Build history of the part. All positions in model axes, mm. A direction names the side the tool comes from. Give positions to 0.01 mm unless a question says otherwise; leave off trailing zeros. Order: outer loops, then holes, each group sorted by start corner. A loop starts at its lowest first (then second) coordinate and runs counter-clockwise, first axis right, second up. Notation, with made-up numbers: (58.25, 49) - (107.25, 49) arc R21 cw to (107.25, 87) - close; hole circle Ø4 at (-25.75, -30.5). An arc over 180 degrees is marked (long way). One line per item, written item: value.
Autodesk Inventor part; units mm, degrees
ref_plane "YZ Plane" through (0, 0, 0) normal (1, 0, 0) x (0, 1, 0)
ref_plane "XZ Plane" through (0, 0, 0) normal (0, 1, 0) x (-1, 0, 0)
ref_plane "XY Plane" through (0, 0, 0) normal (0, 0, 1) x (1, 0, 0)
sketch "Skizze1" plane through (0, 0, 0) normal (0, 0, 1) x (1, 0, 0)
  line L0 (0, 0) -> (0, 47.086)
  line L1 (0, 43.9) -> (-9.5, 43.9)
  line L2 (-9.5, 43.9) -> (-9.5, 22.7)
  line L3 (-9.5, 22.7) -> (-8.5, 22.7)
  line L4 (-8.5, 22.7) -> (-8.5, 0)
  line L5 (-8.5, 0) -> (0, 0)
  dimension "d0" = 19
  dimension "d1" = 17
  dimension "d2" = 43.9
  dimension "d3" = 21.2
revolve "Umdrehung1" add sketch "Skizze1" angle 360 about axis through (0, 0, 0) along (0, 1, 0)
sketch "Skizze2" plane through (0, 0, 0) normal (0, -1, 0) x (1, 0, 0)
  line L0 (5.7629, 1.0144) -> (5, 1.0144)
  line L1 (5, 1.0144) -> (5, -1.0144)
  line L2 (5, -1.0144) -> (5.7629, -1.0144)
  line L3 (5.7629, -1.0144) -> (5.7629, 1.0144)
  point P0 (0, 0)
  point P1 (5.7629, 0)
  dimension "d5" = 5
extrude "Extrusion1" add sketch "Skizze2" along normal blind 5
mirror "Spiegeln1" about plane through (0, 0, 0) normal (1, 0, 0) of "Extrusion1"
sketch "Skizze3" plane through (0, 43.9, 0) normal (0, 1, 0) x (1, 0, 0)
  circle A0 centre (-1.8885, 0) radius 1.75
  circle A1 centre (5.6115, 0) radius 1.75
  point P0 (0, 0)
  dimension "d8" = 7.5
  dimension "d9" = 3.5
extrude "Extrusion2" add sketch "Skizze3" along normal blind 5.5
properties part number "Pumpe_Dummy"
(1) Pull direction X, two halves, no side cores. Call faces 5 (the face through (5.763, -2, 0)), 6 (the face through (6, 49.4, 0)), 7 (the face through (-5, -2, 0)): +X half, -X half, draft (parallel to the pull), parting line (faces both ways), or undercut.
Completed:
face 5: +X half
face 6: draft
face 7: undercut
(2) 3-axis set-ups, long thin cutter, end or side, ignore diameter. For faces 1 (the face through (-5.763, -2, 0)), 2 (the face through (-4.57, 11.191, -7.167)), 3 (the face through (7.23, 46.61, -0.67)), 4 (the face through (5, -2, 0)): which of +Z, -Z, +X, -X, +Y, -Y reach the whole face in a straight line?
Completed:
face 1: +Z, -Z, -X, -Y
face 2: -Y
face 3: +Y
face 4: +Z, -Z, -Y
(3) Drill centre lines: line 1 (Z direction, x = 0, y = 4); line 2 (Y direction, x = -7.75, z = -1.25). Where is each one in solid material? Low to high.
Completed:
line 1: -8.5 to 8.5
line 2: 0 to 43.9
(4) Slice it at C-C, the plane y = 12.5. Give the cut face in (x, z), and give its area (3 significant figures).
Completed:
outline: circle Ø17 at (0, 0)
area: 227 mm²
(5) Slice it at B-B, the plane x = 3.25. Give the cut face in (y, z).
Completed:
outline: (0, -7.85) - (22.7, -7.85) - (22.7, -8.93) - (43.9, -8.93) - (43.9, 8.93) - (22.7, 8.93) - (22.7, 7.85) - (0, 7.85) - close
(6) Pin check, flat tips, straight feed: P1, Ø8, axis at x = 3.5, y = 39, coming from the +Z side; P2, Ø1, axis at y = -2.5, z = 0, coming from the +X side; P3, Ø2, axis at y = -2, z = 0.5, coming from the -X side; P4, Ø0.8, axis at x = -5.5, y = -3, coming from the -Z side. Stop position of each tip, or through.
Completed:
P1: z = 9.5
P2: x = 5.76
P3: x = -5.76
P4: z = -1.01
(7) Slice it at A-A, the plane z = 0. Give the cut face in (x, y), and give its area (3 significant figures).
Completed:
outline: (-9.5, 22.7) - (-8.5, 22.7) - (-8.5, 0) - (-5.76, 0) - (-5.76, -5) - (-5, -5) - (-5, 0) - (5, 0) - (5, -5) - (5.76, -5) - (5.76, 0) - (8.5, 0) - (8.5, 22.7) - (9.5, 22.7) - (9.5, 43.9) - (7.36, 43.9) - (7.36, 49.4) - (3.86, 49.4) - (3.86, 43.9) - (-0.14, 43.9) - (-0.14, 49.4) - (-3.64, 49.4) - (-3.64, 43.9) - (-9.5, 43.9) - close
area: 835 mm²
(8) Slice it at D-D, the plane z = 3.25. Give the cut face in (x, y), and give its area (3 significant figures).
Completed:
outline: (-8.93, 22.7) - (-7.85, 22.7) - (-7.85, 0) - (7.85, 0) - (7.85, 22.7) - (8.93, 22.7) - (8.93, 43.9) - (-8.93, 43.9) - close
area: 735 mm²
